CAD build for the part. Positions are in the model's coordinates, mm. Face numbers are marked on the shaded views. Round coordinates to 2 decimals unless told otherwise and drop trailing zeros. Order: outer loops, then holes, each group sorted by start corner. A loop starts at its lowest first (then second) coordinate and runs counter-clockwise, first axis right, second up. Notation, with made-up numbers: M -28.5,42.5 L -6.5,42.5 A38 cw -6.5,81.5 Z; hole C 77,86.25 d5. An arc over 180 degrees is marked long. Answer as a JSON object with one key per item and string values.
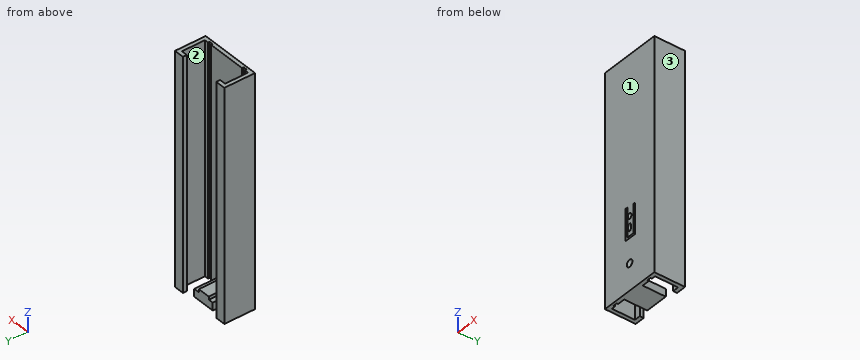
```python
from build123d import *

# Parameters (mm, degrees)
SKETCH_9_W           = 8
SKETCH_9_H           = 4
EXTRUDE_3_DEPTH      = 30
SKETCH_12_W          = 7
SKETCH_12_H          = 3.5
CUT_EXTRUDE_6_DEPTH  = 30
SKETCH_19_W          = 3
SKETCH_19_H          = 1
EXTRUDE_5_DEPTH      = 3
SKETCH_20_W          = 1.605632867
SKETCH_20_H          = 0.400892845
EXTRUDE_6_DEPTH      = 3
SKETCH_22_W          = 0.5
SKETCH_22_H          = 30
CUT_EXTRUDE_7_DEPTH  = 0.2
SKETCH_24_W          = 0.5
SKETCH_24_H          = 30
CUT_EXTRUDE_8_DEPTH  = 0.2
SKETCH_25_R          = 0.457551157
CUT_EXTRUDE_9_DEPTH  = 0.5
SKETCH_26_RX         = 0.496424447
SKETCH_26_RY         = 0.246353064
CUT_EXTRUDE_10_DEPTH = 0.5
SKETCH_27_RX         = 0.374325804
SKETCH_27_RY         = 0.288568922
CUT_EXTRUDE_11_DEPTH = 0.5
SKETCH_28_W          = 0.274311356
SKETCH_28_H          = 4.016178833
CUT_EXTRUDE_12_DEPTH = 0.5
SKETCH_29_W          = 1.237753382
SKETCH_29_H          = 0.3
CUT_EXTRUDE_13_DEPTH = 0.5
SKETCH_31_W          = 0.285973064
SKETCH_31_H          = 3.811928928
CUT_EXTRUDE_14_DEPTH = 0.5
SKETCH_32_W          = 0.8
SKETCH_32_H          = 0.5
EXTRUDE_7_DEPTH      = 30
SKETCH_33_W          = 0.8
SKETCH_33_H          = 0.5
EXTRUDE_8_DEPTH      = 30


with BuildPart() as part:
    # 草圖9 → 填料-伸長3 (new body)
    with BuildSketch(Plane.XY):
        Rectangle(SKETCH_9_W, SKETCH_9_H)
    extrude(amount=EXTRUDE_3_DEPTH)

    # 草圖12 → 除料-伸長6 (cut)
    with BuildSketch(Plane(origin=(0, 0, 0), x_dir=(-1, 0, 0), z_dir=(0, 0, -1))):
        with Locations((0, 0.25)):
            Rectangle(SKETCH_12_W, SKETCH_12_H)
    extrude(amount=-CUT_EXTRUDE_6_DEPTH, mode=Mode.SUBTRACT)

    # 草圖19 → 填料-伸長5 (add)
    with BuildSketch(Plane(origin=(0, -1.5, 0), x_dir=(1, 0, 0), z_dir=(0, 1, 0))):
        with Locations((0, -0.5)):
            Rectangle(SKETCH_19_W, SKETCH_19_H)
    extrude(amount=EXTRUDE_5_DEPTH)

    # 草圖20 → 填料-伸長6 (add)
    with BuildSketch(Plane(origin=(0, -1.5, 0), x_dir=(1, 0, 0), z_dir=(0, 1, 0))):
        with Locations((-0.052553258, -1.200446422)):
            Rectangle(SKETCH_20_W, SKETCH_20_H)
    extrude(amount=EXTRUDE_6_DEPTH)

    # 草圖22 → 除料-伸長7 (cut)
    with BuildSketch(Plane(origin=(0, -1.5, 0), x_dir=(1, 0, 0), z_dir=(0, 1, 0))):
        with Locations((-2.75, -15)):
            Rectangle(SKETCH_22_W, SKETCH_22_H)
    extrude(amount=-CUT_EXTRUDE_7_DEPTH, mode=Mode.SUBTRACT)

    # 草圖24 → 除料-伸長8 (cut)
    with BuildSketch(Plane(origin=(0, -1.5, 0), x_dir=(1, 0, 0), z_dir=(0, 1, 0))):
        with Locations((2.747295887, -15)):
            Rectangle(SKETCH_24_W, SKETCH_24_H)
    extrude(amount=-CUT_EXTRUDE_8_DEPTH, mode=Mode.SUBTRACT)

    # 草圖25 → 除料-伸長9 (cut)
    with BuildSketch(Plane(origin=(0, -1.5, 0), x_dir=(1, 0, 0), z_dir=(0, 1, 0))):
        with Locations(Location((0, -3.470601741, 0), (0, 0, 270))):
            Circle(SKETCH_25_R)
    extrude(amount=-CUT_EXTRUDE_9_DEPTH, mode=Mode.SUBTRACT)

    # 草圖26 → 除料-伸長10 (cut)
    with BuildSketch(Plane(origin=(0, -1.5, 0), x_dir=(1, 0, 0), z_dir=(0, 1, 0))):
        with Locations(Location((0, -8.0522519), (0, 0, 90))):
            Ellipse(SKETCH_26_RX, SKETCH_26_RY)
    extrude(amount=-CUT_EXTRUDE_10_DEPTH, mode=Mode.SUBTRACT)

    # 草圖27 → 除料-伸長11 (cut)
    with BuildSketch(Plane(origin=(0, -1.5, 0), x_dir=(1, 0, 0), z_dir=(0, 1, 0))):
        with Locations(Location((0, -9.480269605), (0, 0, 90))):
            Ellipse(SKETCH_27_RX, SKETCH_27_RY)
    extrude(amount=-CUT_EXTRUDE_11_DEPTH, mode=Mode.SUBTRACT)

    # 草圖28 → 除料-伸長12 (cut)
    with BuildSketch(Plane(origin=(0, -1.5, 0), x_dir=(1, 0, 0), z_dir=(0, 1, 0))):
        with Locations((0.731907804, -8.669902249)):
            Rectangle(SKETCH_28_W, SKETCH_28_H)
    extrude(amount=-CUT_EXTRUDE_12_DEPTH, mode=Mode.SUBTRACT)

    # 草圖29 → 除料-伸長13 (cut)
    with BuildSketch(Plane(origin=(0, -1.5, 0), x_dir=(1, 0, 0), z_dir=(0, 1, 0))):
        with Locations((-0.024124565, -6.811812832)):
            Rectangle(SKETCH_29_W, SKETCH_29_H)
    extrude(amount=-CUT_EXTRUDE_13_DEPTH, mode=Mode.SUBTRACT)

    # 草圖31 → 除料-伸長14 (cut)
    with BuildSketch(Plane(origin=(0, -1.5, 0), x_dir=(1, 0, 0), z_dir=(0, 1, 0))):
        with Locations((-0.500014724, -8.867777296)):
            Rectangle(SKETCH_31_W, SKETCH_31_H)
    extrude(amount=-CUT_EXTRUDE_14_DEPTH, mode=Mode.SUBTRACT)

    # 草圖32 → 填料-伸長7 (add)
    with BuildSketch(Plane(origin=(0, 0, 0), x_dir=(-1, 0, 0), z_dir=(0, 0, -1))):
        with Locations((-3.1, 1.75)):
            Rectangle(SKETCH_32_W, SKETCH_32_H)
    extrude(amount=-EXTRUDE_7_DEPTH)

    # 草圖33 → 填料-伸長8 (add)
    with BuildSketch(Plane(origin=(0, 0, 0), x_dir=(-1, 0, 0), z_dir=(0, 0, -1))):
        with Locations((3.1, 1.75)):
            Rectangle(SKETCH_33_W, SKETCH_33_H)
    extrude(amount=-EXTRUDE_8_DEPTH)


solid = part.part
```
Item 1: Drop flat-ended pins along their axis: pin 1 Ø4 at (x, z) = (0.5, 20) entering from +Y; pin 2 Ø2 at (x, y) = (0, 0) entering from +Z. Give the stop position or say it passes through.
Worked answers:
{"pin 1": "stops at y = -1.5", "pin 2": "stops at z = 1.4"}
Item 2: Saw through at A-A on z = 7.25. List the corners of the cut face in (x, y).
Worked answers:
{"outline": "M -4,-2 L -0.64,-2 L -0.64,-1.5 L -2.5,-1.5 L -2.5,-1.7 L -3,-1.7 L -3,-1.5 L -3.5,-1.5 L -3.5,1.5 L -2.7,1.5 L -2.7,2 L -4,2 Z; M -0.36,-2 L 0.59,-2 L 0.59,-1.5 L -0.36,-1.5 Z; M 0.87,-2 L 4,-2 L 4,2 L 2.7,2 L 2.7,1.5 L 3.5,1.5 L 3.5,-1.5 L 3,-1.5 L 3,-1.7 L 2.5,-1.7 L 2.5,-1.5 L 0.87,-1.5 Z"}
Item 3: Saw through at B-B on z = 4.25. List the corners of the cut face in (x, y).
Worked answers:
{"outline": "M -4,-2 L 4,-2 L 4,2 L 2.7,2 L 2.7,1.5 L 3.5,1.5 L 3.5,-1.5 L 3,-1.5 L 3,-1.7 L 2.5,-1.7 L 2.5,-1.5 L -2.5,-1.5 L -2.5,-1.7 L -3,-1.7 L -3,-1.5 L -3.5,-1.5 L -3.5,1.5 L -2.7,1.5 L -2.7,2 L -4,2 Z"}
Item 4: Wall check: line 1 along X through (y, z) = (0.9, 28.5); line 2 along Y through (x, z) = (-3.25, 22.75); line 3 along Y through (x, z) = (2.75, 14.75). Give the ranges that are in metal, low to high. Write a range as [from, to].
Worked answers:
{"line 1": "x = [-4, -3.5], [3.5, 4]", "line 2": "y = [-2, -1.5], [1.5, 2]", "line 3": "y = [-2, -1.7], [1.5, 2]"}
Item 5: Two-plate mould, pull along Y, no slides. Class the marked faces 1, 2 and 3: released by +Y, released by -Y, zero draft, split by the parting line, or undercut.
Worked answers:
{"face 1": "released by -Y", "face 2": "undercut", "face 3": "zero draft"}
